```python
from build123d import *

# Parameters (mm, degrees)
SKETCH1_R           = 1
BOSS_EXTRUDE1_DEPTH = 55


with BuildPart() as part:
    # Sketch1 → Boss-Extrude1 (new body, symmetric)
    with BuildSketch(Plane.XY):
        with BuildLine():
            ThreePointArc((-6, 1.25), (-5.926776695, 1.073223305), (-5.75, 1))
            Line((-5.75, 1), (-4.75, 1))
            ThreePointArc((-4.75, 1), (-4.573223305, 1.073223305), (-4.5, 1.25))
            Line((-4.5, 1.25), (-4.5, 2.835786438))
            ThreePointArc((-4.5, 2.835786438), (-4.345670858, 3.066756321), (-4.073223305, 3.012563133))
            Line((-4.073223305, 3.012563133), (-2.573223305, 1.512563133))
            ThreePointArc((-2.573223305, 1.512563133), (-2.519030117, 1.431457296), (-2.5, 1.335786438))
            Line((-2.5, 1.335786438), (-2.5, -1.335786438))
            ThreePointArc((-2.5, -1.335786438), (-2.519030117, -1.431457296), (-2.573223305, -1.512563133))
            Line((-2.573223305, -1.512563133), (-4.073223305, -3.012563133))
            ThreePointArc((-4.073223305, -3.012563133), (-4.345670858, -3.066756321), (-4.5, -2.835786438))
            Line((-4.5, -2.835786438), (-4.5, -1.25))
            ThreePointArc((-4.5, -1.25), (-4.573223305, -1.073223305), (-4.75, -1))
            Line((-4.75, -1), (-5.75, -1))
            ThreePointArc((-5.75, -1), (-5.926776695, -1.073223305), (-6, -1.25))
            Line((-6, -1.25), (-6, -5.75))
            ThreePointArc((-6, -5.75), (-5.926776695, -5.926776695), (-5.75, -6))
            Line((-5.75, -6), (-1.25, -6))
            ThreePointArc((-1.25, -6), (-1.073223305, -5.926776695), (-1, -5.75))
            Line((-1, -5.75), (-1, -4.75))
            ThreePointArc((-1, -4.75), (-1.073223305, -4.573223305), (-1.25, -4.5))
            Line((-1.25, -4.5), (-2.835786438, -4.5))
            ThreePointArc((-2.835786438, -4.5), (-3.066756321, -4.345670858), (-3.012563133, -4.073223305))
            Line((-3.012563133, -4.073223305), (-1.512563133, -2.573223305))
            ThreePointArc((-1.512563133, -2.573223305), (-1.431457296, -2.519030117), (-1.335786438, -2.5))
            Line((-1.335786438, -2.5), (1.335786438, -2.5))
            ThreePointArc((1.335786438, -2.5), (1.431457296, -2.519030117), (1.512563133, -2.573223305))
            Line((1.512563133, -2.573223305), (3.012563133, -4.073223305))
            ThreePointArc((3.012563133, -4.073223305), (3.066756321, -4.345670858), (2.835786438, -4.5))
            Line((2.835786438, -4.5), (1.25, -4.5))
            ThreePointArc((1.25, -4.5), (1.073223305, -4.573223305), (1, -4.75))
            Line((1, -4.75), (1, -5.75))
            ThreePointArc((1, -5.75), (1.073223305, -5.926776695), (1.25, -6))
            Line((1.25, -6), (5.75, -6))
            ThreePointArc((5.75, -6), (5.926776695, -5.926776695), (6, -5.75))
            Line((6, -5.75), (6, -1.25))
            ThreePointArc((6, -1.25), (5.926776695, -1.073223305), (5.75, -1))
            Line((5.75, -1), (4.75, -1))
            ThreePointArc((4.75, -1), (4.573223305, -1.073223305), (4.5, -1.25))
            Line((4.5, -1.25), (4.5, -2.835786438))
            ThreePointArc((4.5, -2.835786438), (4.345670858, -3.066756321), (4.073223305, -3.012563133))
            Line((4.073223305, -3.012563133), (2.573223305, -1.512563133))
            ThreePointArc((2.573223305, -1.512563133), (2.519030117, -1.431457296), (2.5, -1.335786438))
            Line((2.5, -1.335786438), (2.5, 1.335786438))
            ThreePointArc((2.5, 1.335786438), (2.519030117, 1.431457296), (2.573223305, 1.512563133))
            Line((2.573223305, 1.512563133), (4.073223305, 3.012563133))
            ThreePointArc((4.073223305, 3.012563133), (4.345670858, 3.066756321), (4.5, 2.835786438))
            Line((4.5, 2.835786438), (4.5, 1.25))
            ThreePointArc((4.5, 1.25), (4.573223305, 1.073223305), (4.75, 1))
            Line((4.75, 1), (5.75, 1))
            ThreePointArc((5.75, 1), (5.926776695, 1.073223305), (6, 1.25))
            Line((6, 1.25), (6, 5.75))
            ThreePointArc((6, 5.75), (5.926776695, 5.926776695), (5.75, 6))
            Line((5.75, 6), (1.25, 6))
            ThreePointArc((1.25, 6), (1.073223305, 5.926776695), (1, 5.75))
            Line((1, 5.75), (1, 4.75))
            ThreePointArc((1, 4.75), (1.073223305, 4.573223305), (1.25, 4.5))
            Line((1.25, 4.5), (2.835786438, 4.5))
            ThreePointArc((2.835786438, 4.5), (3.066756321, 4.345670858), (3.012563133, 4.073223305))
            Line((3.012563133, 4.073223305), (1.439339828, 2.5))
            Line((1.439339828, 2.5), (-1.335786438, 2.5))
            ThreePointArc((-1.335786438, 2.5), (-1.431457296, 2.519030117), (-1.512563133, 2.573223305))
            Line((-1.512563133, 2.573223305), (-3.012563133, 4.073223305))
            ThreePointArc((-3.012563133, 4.073223305), (-3.066756321, 4.345670858), (-2.835786438, 4.5))
            Line((-2.835786438, 4.5), (-1.25, 4.5))
            ThreePointArc((-1.25, 4.5), (-1.073223305, 4.573223305), (-1, 4.75))
            Line((-1, 4.75), (-1, 5.75))
            ThreePointArc((-1, 5.75), (-1.073223305, 5.926776695), (-1.25, 6))
            Line((-1.25, 6), (-5.75, 6))
            ThreePointArc((-5.75, 6), (-5.926776695, 5.926776695), (-6, 5.75))
            Line((-6, 5.75), (-6, 1.25))
        make_face()
        Circle(SKETCH1_R, mode=Mode.SUBTRACT)
    extrude(amount=BOSS_EXTRUDE1_DEPTH, both=True)


solid = part.part
```
Here's how the part is built. I have some questions about the finished solid (model axes, mm). A direction names the side the tool comes from. Give positions to 0.01 mm unless a question says otherwise; leave off trailing zeros. Order: outer loops, then holes, each group sorted by start corner. A loop starts at its lowest first (then second) coordinate and runs counter-clockwise, first axis right, second up. Notation, with made-up numbers: (56.5, 83.25) - (61.5, 83.25) arc R29 cw to (61.5, 104.25) - close; hole circle Ø10 at (-34, 53). An arc over 180 degrees is marked (long way). Answer as a JSON object with one key per item and string values. Group by question number.
Item 1: If we mould it in two halves opening along Y, with no side actions, what happens to faces 3 (the flat face through (2.5, 0, 1)), 4 (the flat face through (6, 3, 1)), 5 (the flat face through (3, -6, 1))? For each: pulls with the +Y half, pulls with the -Y half, needs draft (parallel to the pull), parting line crosses it, or undercut.
Item 2: Please list where these lines run through material, in increasing order: probe 1 along Y at (x, z) = (1.5, -31); probe 2 along Y at (x, z) = (0, -1); probe 3 along X at (y, z) = (5.25, 49.5).
Item 3: Which directions (+Z, -Z, +X, -X, +Y, -Y) give clear straight access to the entire face, cutting with the end or side of a thin tool? Please do faces 1 (the flat face through (-3, 6, 1)), 2 (the flat face through (0, -2.5, 1)).
Item 4: If we section it at A-A on y = 0: Please give me the cut outline in (x, z), and give its area (3 significant figures).
Result set:
{
 "1": {"face 3": "undercut", "face 4": "needs draft", "face 5": "pulls with the -Y half"},
 "2": {"probe 1": "-6 to -4.5, -2.56 to 2.56, 4.5 to 6", "probe 2": "-2.5 to -1, 1 to 2.5", "probe 3": "-6 to -1, 1 to 6"},
 "3": {"face 1": "+Z, -Z, +X, -X, +Y", "face 2": "+Z, -Z"},
 "4": {"outline": "(-2.5, -55) - (-1, -55) - (-1, 55) - (-2.5, 55) - close; (1, -55) - (2.5, -55) - (2.5, 55) - (1, 55) - close", "area": "330 mm²"}
}
